Geometry: final body of the model. Coordinates: model frame, mm. Coordinates: 2 decimals unless noted, no trailing zeros. Order: outer loops, then holes, each group sorted by start corner. A loop starts at its lowest first (then second) coordinate and runs counter-clockwise, first axis right, second up. Notation, with made-up numbers: M 21.25,35 L 69.25,35 A22 ccw 69.25,56 Z; hole C -15,51 d6. An arc over 180 degrees is marked long. Use CSV: the item, a comma, the result in double quotes. Start each with the question number.
1. Section query B-B on x = 45. Return the cut outline in (y, z), and give its area (3 significant figures).
2. Section query D-D on z = -49. Return the cut outline in (x, y).
3. First-contact query: P1, Ø7.5, axis at x = -45, z = 16.5, coming from the +Y side. Flat tip, straight axial feed; report the tip coordinate or a pass-through.
4. Section query A-A on z = 16.5. Return the cut outline in (x, y).
5. Material intervals for line 1 (Z direction, x = 45, y = -1.25); line 2 (Z direction, x = -12, y = 1.3); line 3 (X direction, y = -1.7, z = 36.5), sorted ascending.
6. Section query C-C on y = 1.05. Return the cut outline in (x, z).
from build123d import *

# Parameters (mm, degrees)
RESSALTO_EXTRUS_O1_DEPTH  = 2
CORTE_EXTRUS_O1_DEPTH     = 167.217478022
PADR_O_LINEAR1_COUNT      = 2
PADR_O_LINEAR1_PITCH      = 90
PADR_O_LINEAR1_COUNT_DIR2 = 2
PADR_O_LINEAR1_PITCH_DIR2 = 20


with BuildPart() as part:
    # Esboço2 → Ressalto-extrusão1 (new, symmetric)
    with BuildSketch(Plane(origin=(0, 0, 0), x_dir=(1, 0, 0), z_dir=(0, 1, 0))):
        with BuildLine():
            Line((75, 71.5), (-75, 71.5))
            ThreePointArc((-75, 71.5), (-128.033008589, 49.533008589), (-150, -3.5))
            Line((-150, -3.5), (-150, -41.5))
            ThreePointArc((-150, -41.5), (-141.213203436, -62.713203436), (-120, -71.5))
            Line((-120, -71.5), (120, -71.5))
            ThreePointArc((120, -71.5), (141.213203436, -62.713203436), (150, -41.5))
            Line((150, -41.5), (150, -3.5))
            ThreePointArc((150, -3.5), (128.033008589, 49.533008589), (75, 71.5))
        make_face()
    extrude(amount=RESSALTO_EXTRUS_O1_DEPTH, both=True)

    # Esboço3 → Corte-extrusão1 (cut, through all)
    with BuildSketch(Plane(origin=(0, 2, 0), x_dir=(1, 0, 0), z_dir=(0, 1, 0))):
        with BuildLine():
            Line((-77.5, 53.5), (77.5, 53.5))
            ThreePointArc((77.5, 53.5), (82.5, 48.5), (77.5, 43.5))
            Line((77.5, 43.5), (-77.5, 43.5))
            ThreePointArc((-77.5, 43.5), (-82.5, 48.5), (-77.5, 53.5))
        make_face()
        with BuildLine():
            Line((-97.5, 33.5), (97.5, 33.5))
            ThreePointArc((97.5, 33.5), (102.5, 28.5), (97.5, 23.5))
            Line((97.5, 23.5), (-97.5, 23.5))
            ThreePointArc((-97.5, 23.5), (-102.5, 28.5), (-97.5, 33.5))
        make_face()
        with BuildLine():
            Line((-120, 13.5), (120, 13.5))
            ThreePointArc((120, 13.5), (125, 8.5), (120, 3.5))
            Line((120, 3.5), (-120, 3.5))
            ThreePointArc((-120, 3.5), (-125, 8.5), (-120, 13.5))
        make_face()
    extrude(amount=-CORTE_EXTRUS_O1_DEPTH, mode=Mode.SUBTRACT)

    # Esboço5 → Escareado para parafuso com cabeça escareada elevada de M61 (revolve, cut)
    with BuildSketch(Plane(origin=(-45, 2, 36.5), x_dir=(0, 0, 1), z_dir=(1, 0, 0))):
        Polygon((0, 0), (0, 4), (3.3, 4), (3.3, 3), (6.3, 0), align=None)
    escareado_para_parafuso_com_cabe_a_escar = revolve(axis=Axis((-45, 8.35, 36.5), (0, -1, 0)), mode=Mode.SUBTRACT)

    # Padrão linear1: Escareado para parafuso com cabe_a escar 2 × 2
    with Locations(*[(i * PADR_O_LINEAR1_PITCH, 0, -j * PADR_O_LINEAR1_PITCH_DIR2) for i in range(PADR_O_LINEAR1_COUNT) for j in range(PADR_O_LINEAR1_COUNT_DIR2) if (i, j) != (0, 0)]):
        add(escareado_para_parafuso_com_cabe_a_escar, mode=Mode.SUBTRACT)


solid = part.part
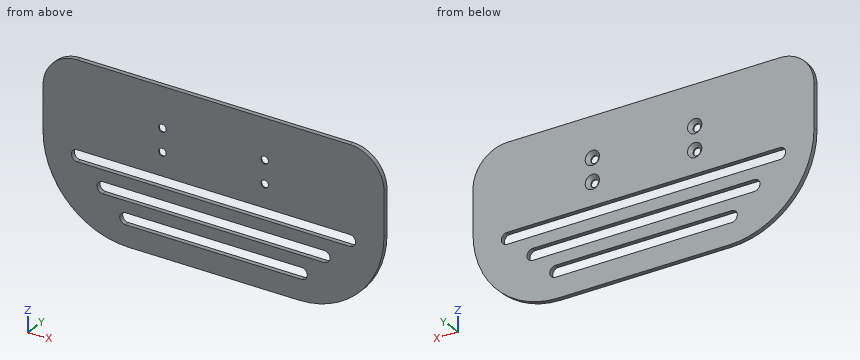
Results list:
1,outline,"M -2,-71.5 L 2,-71.5 L 2,-53.5 L -2,-53.5 Z; M -2,-43.5 L 2,-43.5 L 2,-33.5 L -2,-33.5 Z; M -2,-23.5 L 2,-23.5 L 2,-13.5 L -2,-13.5 Z; M -2,-3.5 L 2,-3.5 L 2,10.2 L -1,13.2 L -2,13.2 Z; M -2,19.8 L -1,19.8 L 2,22.8 L 2,30.2 L -1,33.2 L -2,33.2 Z; M -2,39.8 L -1,39.8 L 2,42.8 L 2,71.5 L -2,71.5 Z"
1,area,"381 mm²"
2,outline,"M -128.56,-2 L -82.47,-2 L -82.47,2 L -128.56,2 Z; M 82.47,-2 L 128.56,-2 L 128.56,2 L 82.47,2 Z"
3,P1,"stops at y = -0.55"
4,outline,"M -150,-2 L -48.3,-2 L -48.3,-1 L -51.3,2 L -150,2 Z; M -41.7,-2 L 41.7,-2 L 41.7,-1 L 38.7,2 L -38.7,2 L -41.7,-1 Z; M 48.3,-2 L 150,-2 L 150,2 L 51.3,2 L 48.3,-1 Z"
5,line 1,"z = -71.5 to -53.5, -43.5 to -33.5, -23.5 to -13.5, -3.5 to 13.2, 19.8 to 33.2, 39.8 to 71.5"
5,line 2,"z = -71.5 to -53.5, -43.5 to -33.5, -23.5 to -13.5, -3.5 to 71.5"
5,line 3,"x = -150 to -48.3, -41.7 to 41.7, 48.3 to 150"
6,outline,"M -150,3.5 A75 ccw -75,-71.5 L 75,-71.5 A75 ccw 150,3.5 L 150,41.5 A30 ccw 120,71.5 L -120,71.5 A30 ccw -150,41.5 Z; hole M -120,-13.5 L 120,-13.5 A5 ccw 120,-3.5 L -120,-3.5 A5 ccw Z; hole M -97.5,-33.5 L 97.5,-33.5 A5 ccw 97.5,-23.5 L -97.5,-23.5 A5 ccw Z; hole M -77.5,-53.5 L 77.5,-53.5 A5 ccw 77.5,-43.5 L -77.5,-43.5 A5 ccw Z; hole C -45,16.5 d10.7; hole C -45,36.5 d10.7; hole C 45,16.5 d10.7; hole C 45,36.5 d10.7"
